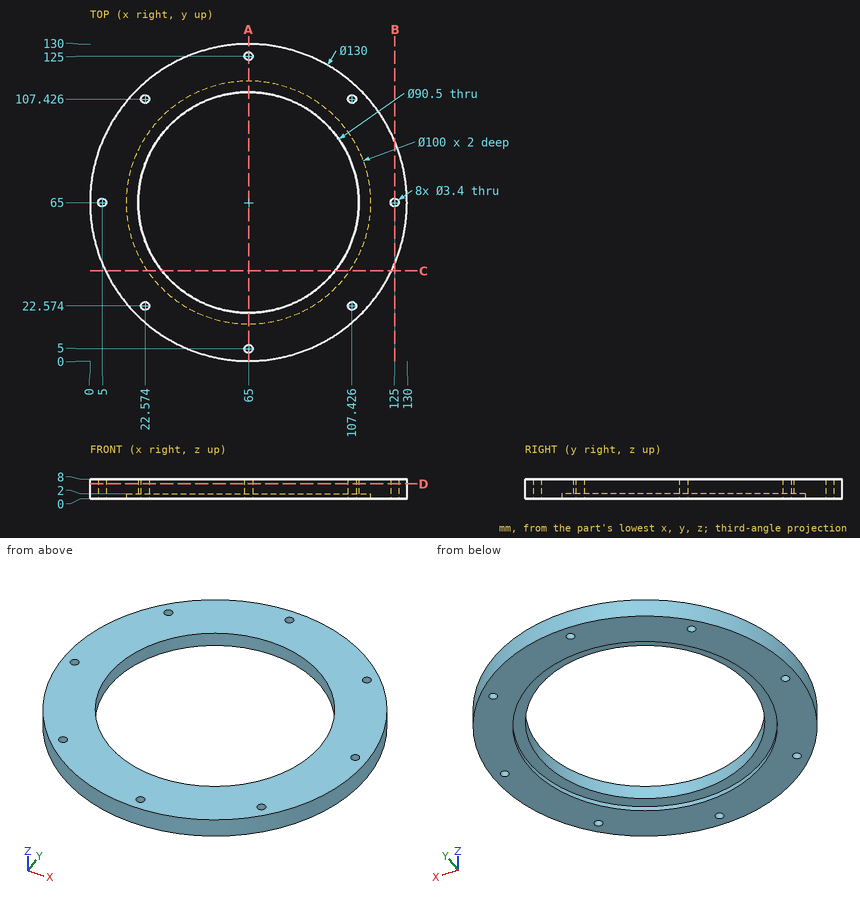
The figure shows three views and two pictorial views of one solid part (mm, origin at its lowest corner). Answer the questions. Round coordinates to 2 decimals unless told otherwise and drop trailing zeros. Order: outer loops, then holes, each group sorted by start corner. A loop starts at its lowest first (then second) coordinate and runs counter-clockwise, first axis right, second up. Notation, with made-up numbers: M 81.25,-31 L 139.25,-31 A20 ccw 139.25,-7 Z; hole C 13,31 d11. An arc over 180 degrees is marked long. Put each result on its own line as item: value. Start each with the question number.
Q1. Section C-C, the plane y = 37 is taken. Write down the section's boundary in (x, z) (1 decimal).
Q2. Section D-D, the plane z = 6 is taken. Give the number of separate pieces and of enclosed holes in the cut face, and give its area (3 significant figures).
Q3. Straight lines are drawn through the part: L1, parallel to Y at x = 65, z = 5.55; L2, parallel to X at y = 66, z = 4.5 (1 decimal); L3, parallel to X at y = 23, z = 1.25 (1 decimal). For each, find the intervals that lie inside material, in ascending order. Write a range as [from, to].
Q4. Section A-A, the plane x = 65 is taken. Write down the section's boundary in (y, z).
Q5. Flat-ended cylindrical pins translate along their axes: pin 1 (1.5 mm diameter, centred on x = 39.5, z = 6, fed in from +Y); pin 2 (3 mm diameter, centred on y = 16.5, z = 6.5, fed in from +X); pin 3 (1.5 mm diameter, centred on y = 95, z = 2, fed in from -X). Find the tip coordinate at first contact, or state that the pin passes through.
Q6. Section B-B, the plane x = 125 is taken. Write down the section's boundary in (y, z).
Findings below:
1. outline: M 6.3,0 L 23.6,0 L 23.6,2 L 29.5,2 L 29.5,8 L 6.3,8 Z; M 100.5,2 L 106.4,2 L 106.4,0 L 123.7,0 L 123.7,8 L 100.5,8 Z
2. separate pieces: 1
2. enclosed holes: 9
2. area: 6,770 mm^2
3. L1: y = [0, 3.3], [6.7, 19.75], [110.25, 123.3], [126.7, 130]
3. L2: x = [0, 3.6], [6.4, 19.8], [110.2, 123.6], [126.4, 130]
3. L3: x = [15.4, 20.9], [24.2, 37.9], [92.1, 105.8], [109.1, 114.6]
4. outline: M 0,0 L 3.3,0 L 3.3,8 L 0,8 Z; M 6.7,0 L 15,0 L 15,2 L 19.75,2 L 19.75,8 L 6.7,8 Z; M 110.25,2 L 115,2 L 115,0 L 123.3,0 L 123.3,8 L 110.25,8 Z; M 126.7,0 L 130,0 L 130,8 L 126.7,8 Z
5. pin 1: stops at y = 125.1
5. pin 2: stops at x = 109.9
5. pin 3: stops at x = 6.95
6. outline: M 40,0 L 63.3,0 L 63.3,8 L 40,8 Z; M 66.7,0 L 90,0 L 90,8 L 66.7,8 Z
